Read the model definition and answer for the solid it produces. Units are mm, in the model's axes. Face numbers are marked on the shaded views. A direction names the side the tool comes from. Coordinates: 2 decimals unless noted, no trailing zeros. Order: outer loops, then holes, each group sorted by start corner. A loop starts at its lowest first (then second) coordinate and runs counter-clockwise, first axis right, second up. Notation, with made-up numbers: (70.25, 57) - (81.25, 57) arc R14 ccw to (81.25, 71) - close; hole circle Ø1 at (51, -21). An arc over 180 degrees is marked (long way). Use one line per item in the form item = value.
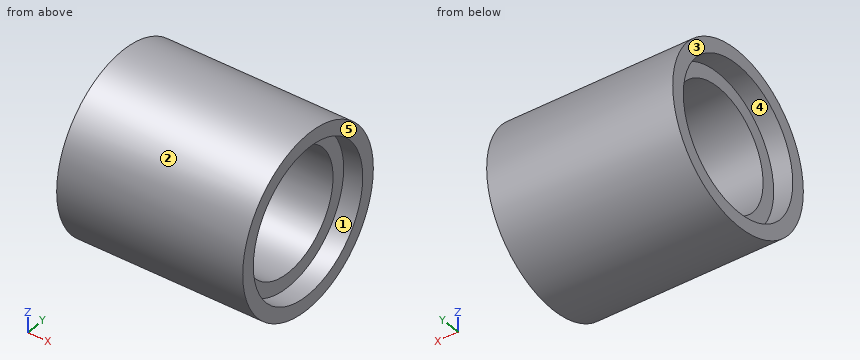
```python
from build123d import *

# Parameters (mm, degrees)
SKETCH_1_R          = 3.7
EXTRUDE_1_DEPTH     = 3.9
SKETCH_2_R          = 2.5
CUT_EXTRUDE_1_DEPTH = 10.392550239
SKETCH_2_3_R        = 3.1
SKETCH_2_3_R_2      = 2.5
CUT_EXTRUDE_2_DEPTH = 0.8


with BuildPart() as part:
    # 草图1 → 凸台-拉伸1 (new, symmetric)
    with BuildSketch(Plane(origin=(0, 0, 0), x_dir=(0, 0, -1), z_dir=(1, 0, 0))):
        Circle(SKETCH_1_R)
    extrude(amount=EXTRUDE_1_DEPTH, both=True)

    # 草图2 → 切除-拉伸1 (cut, through all)
    with BuildSketch(Plane(origin=(3.9, 0, 0), x_dir=(0, 0, -1), z_dir=(1, 0, 0))):
        Circle(SKETCH_2_R)
    extrude(amount=-CUT_EXTRUDE_1_DEPTH, mode=Mode.SUBTRACT)

    # 草图2<3> → 切除-拉伸2 (cut)
    with BuildSketch(Plane(origin=(3.9, 0, 0), x_dir=(0, 0, -1), z_dir=(1, 0, 0))):
        Circle(SKETCH_2_3_R)
        Circle(SKETCH_2_3_R_2, mode=Mode.SUBTRACT)
    cut_extrude_2 = extrude(amount=-CUT_EXTRUDE_2_DEPTH, mode=Mode.SUBTRACT)

    # 镜向1: 切除-拉伸2 across plane
    add(cut_extrude_2.mirror(Plane(origin=(0, 0, 0), x_dir=(0, 0, 1), z_dir=(1, 0, 0))), mode=Mode.SUBTRACT)


solid = part.part
```
(1) Section B-B, the plane y = -2 is taken. Write down the section's boundary in (x, z), then the cut area to 3 significant figures.
Answer list:
outline = (-3.9, -3.11) - (3.9, -3.11) - (3.9, -2.37) - (3.1, -2.37) - (3.1, -1.5) - (-3.1, -1.5) - (-3.1, -2.37) - (-3.9, -2.37) - close; (-3.9, 2.37) - (-3.1, 2.37) - (-3.1, 1.5) - (3.1, 1.5) - (3.1, 2.37) - (3.9, 2.37) - (3.9, 3.11) - (-3.9, 3.11) - close
area = 22.4 mm2
(2) Which of the six approach directions +Z, -Z, +X, -X, +Y, -Y give full straight-line access (tool end or side, diameter ignored) to the marked faces 4 and 5?
Answer list:
face_4 = -X
face_5 = +Z, -Z, +X, +Y, -Y
(3) Section A-A, the plane z = 0 is taken. Write down the section's boundary in (x, y), then the cut area to 3 significant figures.
Answer list:
outline = (-3.9, -3.7) - (3.9, -3.7) - (3.9, -3.1) - (3.1, -3.1) - (3.1, -2.5) - (-3.1, -2.5) - (-3.1, -3.1) - (-3.9, -3.1) - close; (-3.9, 3.1) - (-3.1, 3.1) - (-3.1, 2.5) - (3.1, 2.5) - (3.1, 3.1) - (3.9, 3.1) - (3.9, 3.7) - (-3.9, 3.7) - close
area = 16.8 mm2
(4) Section C-C, the plane x = -0.5 is taken. Write down the section's boundary in (y, z), then the cut area to 3 significant figures.
Answer list:
outline = circle Ø7.4 at (0, 0); hole circle Ø5 at (0, 0)
area = 23.4 mm2
(5) Straight lines are drawn through the part: L1, parallel to Y at x = 3.4, z = 0; L2, parallel to Y at x = 0, z = 0; L3, parallel to Z at x = -2, y = -0.5. For each, find the intervals that lie inside material, in ascending order.
Answer list:
L1 = -3.7 to -3.1, 3.1 to 3.7
L2 = -3.7 to -2.5, 2.5 to 3.7
L3 = -3.67 to -2.45, 2.45 to 3.67
(6) The mould has two halves that part along Y. Classify the marked faces 1, 2 and 3: +Y half, -Y half, draft (parallel to the pull), parting line (faces both ways), or undercut.
Answer list:
face_1 = undercut
face_2 = parting line
face_3 = draft
(7) Given pin 1 Ø1 at (x, z) = (1, 2.5) entering from -Y; pin 2 Ø1.9 at (y, z) = (1, -1) entering from -X; pin 3 Ø2 at (y, z) = (-2, -0.5) entering from +X, each flat-ended and moving along its own axis, determine where each tip first touches the part or whether it passes through.
Answer list:
pin_1 = -3.11
pin_2 = through
pin_3 = 3.1
